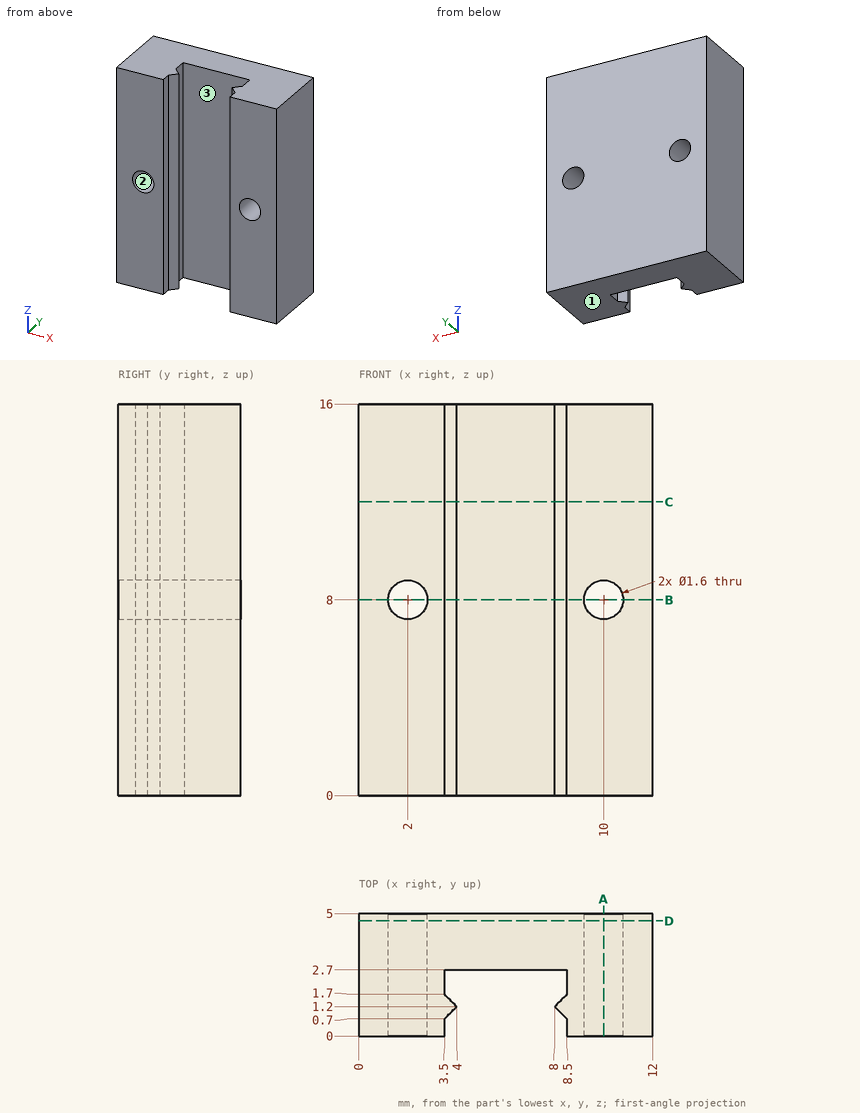
Study the drawing (mm; zero at the part's minimum x, y, z) and answer. Give positions to 0.01 mm unless a question says otherwise; leave off trailing zeros. Order: outer loops, then holes, each group sorted by start corner. A loop starts at its lowest first (then second) coordinate and runs counter-clockwise, first axis right, second up.
1) Find section D-D on y = 4.7. Write down the section's boundary in (x, z), then the cut area to 3 significant figures.
Reported:
outline: (0, 0) - (12, 0) - (12, 16) - (0, 16) - close; hole circle Ø1.6 at (2, 8); hole circle Ø1.6 at (10, 8)
area: 188 mm2
2) Find section C-C on z = 12. Write down the section's boundary in (x, y), then the cut area to 3 significant figures.
Reported:
outline: (0, 0) - (3.5, 0) - (3.5, 0.7) - (4, 1.2) - (3.5, 1.7) - (3.5, 2.7) - (8.5, 2.7) - (8.5, 1.7) - (8, 1.2) - (8.5, 0.7) - (8.5, 0) - (12, 0) - (12, 5) - (0, 5) - close
area: 47.0 mm2
3) Determine the mould class of the marked faces 1, 2 and 3 for opening direction Z: pulls with the +Z half, pulls with the -Z half, needs draft (parallel to the pull), parting line crosses it, or undercut.
Reported:
face 1: pulls with the -Z half
face 2: undercut
face 3: needs draft
4) Consider line 1 along X through (y, z) = (3.7, 8); line 2 along X through (y, z) = (2.35, 8); line 3 along X through (y, z) = (1.9, 1.5). Determine where each line is inside the solid, lowest interval first.
Reported:
line 1: x = 0 to 1.2, 2.8 to 9.2, 10.8 to 12
line 2: x = 0 to 1.2, 2.8 to 3.5, 8.5 to 9.2, 10.8 to 12
line 3: x = 0 to 3.5, 8.5 to 12
5) Find section B-B on z = 8. Write down the section's boundary in (x, y).
Reported:
outline: (0, 0) - (1.2, 0) - (1.2, 5) - (0, 5) - close; (2.8, 0) - (3.5, 0) - (3.5, 0.7) - (4, 1.2) - (3.5, 1.7) - (3.5, 2.7) - (8.5, 2.7) - (8.5, 1.7) - (8, 1.2) - (8.5, 0.7) - (8.5, 0) - (9.2, 0) - (9.2, 5) - (2.8, 5) - close; (10.8, 0) - (12, 0) - (12, 5) - (10.8, 5) - close
6) Given P1, Ø1.4, axis at x = 10, z = 8, coming from the -Y side; P2, Ø1.5, axis at x = 7.5, z = 12, coming from the -Y side, each flat-ended and moving along its own axis, determine where each tip first touches the part or whether it passes through.
Reported:
P1: passes through
P2: stops at y = 0.95
7) Find section A-A on x = 10. Write down the section's boundary in (y, z), then the cut area to 3 significant figures.
Reported:
outline: (0, 0) - (5, 0) - (5, 7.2) - (0, 7.2) - close; (0, 8.8) - (5, 8.8) - (5, 16) - (0, 16) - close
area: 72.0 mm2
